The listing builds one solid part. Answer for the finished solid, in the listing's coordinates (mm). Give positions to 0.01 mm unless a question says otherwise; leave off trailing zeros. Order: outer loops, then holes, each group sorted by start corner. A loop starts at its lowest first (then second) coordinate and runs counter-clockwise, first axis right, second up.
```python
from build123d import *

# Parameters (mm, degrees)
BOSS_EXTRUDE1_DEPTH    = 800
CAP_SCREW1_D           = 3.5
CAP_SCREW1_CBORE_D     = 6
CAP_SCREW1_CBORE_DEPTH = 4.5
SCALE_1_SCALE          = 1.7


with BuildPart() as part:
    # Sketch1 → Boss-Extrude1 (new body)
    with BuildSketch(Plane(origin=(-20, 0, 0), x_dir=(0, 0, -1), z_dir=(1, 0, 0))):
        with BuildLine():
            Line((-5.692330317, 12.5), (5.692330317, 12.5))
            Line((5.692330317, 12.5), (6.192330317, 12))
            ThreePointArc((6.192330317, 12), (6.706274607, 11.346743741), (7.5, 11.1))
            Line((7.5, 11.1), (7.5, 9.5))
            ThreePointArc((7.5, 9.5), (6.1, 8.1), (7.5, 6.7))
            Line((7.5, 6.7), (7.5, 1))
            Line((7.5, 1), (6.5, 0))
            Line((6.5, 0), (-6.5, 0))
            Line((-6.5, 0), (-7.5, 1))
            Line((-7.5, 1), (-7.5, 6.7))
            ThreePointArc((-7.5, 6.7), (-6.1, 8.1), (-7.5, 9.5))
            Line((-7.5, 9.5), (-7.5, 11.1))
            ThreePointArc((-7.5, 11.1), (-6.706274607, 11.346743741), (-6.192330317, 12))
            Line((-6.192330317, 12), (-5.692330317, 12.5))
        make_face()
    extrude(amount=BOSS_EXTRUDE1_DEPTH)

    # Cap Screw1 (through all)
    with Locations(Plane(origin=(0, 12.5, 0), x_dir=(1, 0, 0), z_dir=(0, 1, 0))):
        with Locations((0, 0), (60, 0), (120, 0), (180, 0), (240, 0), (300, 0), (360, 0), (420, 0), (480, 0), (540, 0), (600, 0), (660, 0), (720, 0)):
            CounterBoreHole(CAP_SCREW1_D / 2, CAP_SCREW1_CBORE_D / 2, CAP_SCREW1_CBORE_DEPTH)


with BuildPart() as part_1:
    # 缩放比例1: scaled about (0, 0, 0)
    add(part.part.scale(SCALE_1_SCALE))


solid = part_1.part
```
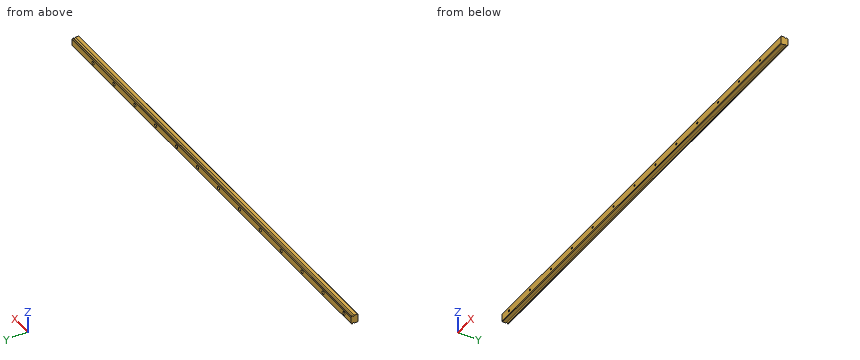
1) Straight lines are drawn through the part: probe 1 along Z at (x, y) = (611, 18.5); probe 2 along Z at (x, y) = (714, 7) (3 decimals); probe 3 along Z at (x, y) = (895.5, 19.75). For each, find the intervals that lie inside material, in ascending order.
Geometry says:
probe 1: z = -12.75 to -5, 5 to 12.75
probe 2: z = -12.75 to -2.975, 2.975 to 12.75
probe 3: z = -10.9 to 10.9
2) Given P1, Ø8, axis at x = 612, z = 0, coming from the +Y side, flat-ended and moving along its own axis, determine where the tip first touches the part or whether it passes through.
Geometry says:
P1: stops at y = 13.6
3) Find section A-A (x = 468). Write down the section's boundary in (y, z).
Geometry says:
outline: (0, -11.05) - (1.7, -12.75) - (11.39, -12.75) arc R2.38 cw to (16.15, -12.75) - (18.87, -12.75) arc R2.38 cw to (20.4, -10.53) - (21.25, -9.68) - (21.25, 9.68) - (20.4, 10.53) arc R2.38 cw to (18.87, 12.75) - (16.15, 12.75) arc R2.38 cw to (11.39, 12.75) - (1.7, 12.75) - (0, 11.05) - close
